Part print with two shaded views. Sizes in mm from the minimum x, y, z corner. Round coordinates to 2 decimals unless told otherwise and drop trailing zeros. Loops run counter-clockwise (first coordinate to the right, second up) from the corner with the lowest first, then second, coordinate; pieces in that order, holes last. Notation, with made-up numbers: M -27,46.25 L 18,46.25 A27 ccw 18,84.25 Z; hole C -31.75,34.25 d9. An arc over 180 degrees is marked long. Answer as CSV lines item,"result". Start each with the question number.
Item 1: Band-saw the part on A-A (x = 19.05). Give the cut face in (y, z), and give its area (3 significant figures).
Item 2: Mould opens along Z. For the marked faces 1, 2, 3 and 4 say: pulls with the +Z half, pulls with the -Z half, needs draft (parallel to the pull), parting line crosses it, or undercut.
Item 3: Band-saw the part on C-C (y = 3.5). Give the cut face in (x, z).
Item 4: Drop flat-ended pins along their axis: pin 1 Ø5 at (x, z) = (34.05, 34.05) entering from -Y; pin 2 Ø2 at (y, z) = (3.5, 15.5) entering from +X. Give the stop position or say it passes through.
Item 5: Wall check: line 1 (X direction, y = 5, z = 49.05); line 2 (X direction, y = 5, z = 9.5); line 3 (Z direction, x = 5, y = 1.25) (1 decimal). Give the ranges that are in metal, low to high.
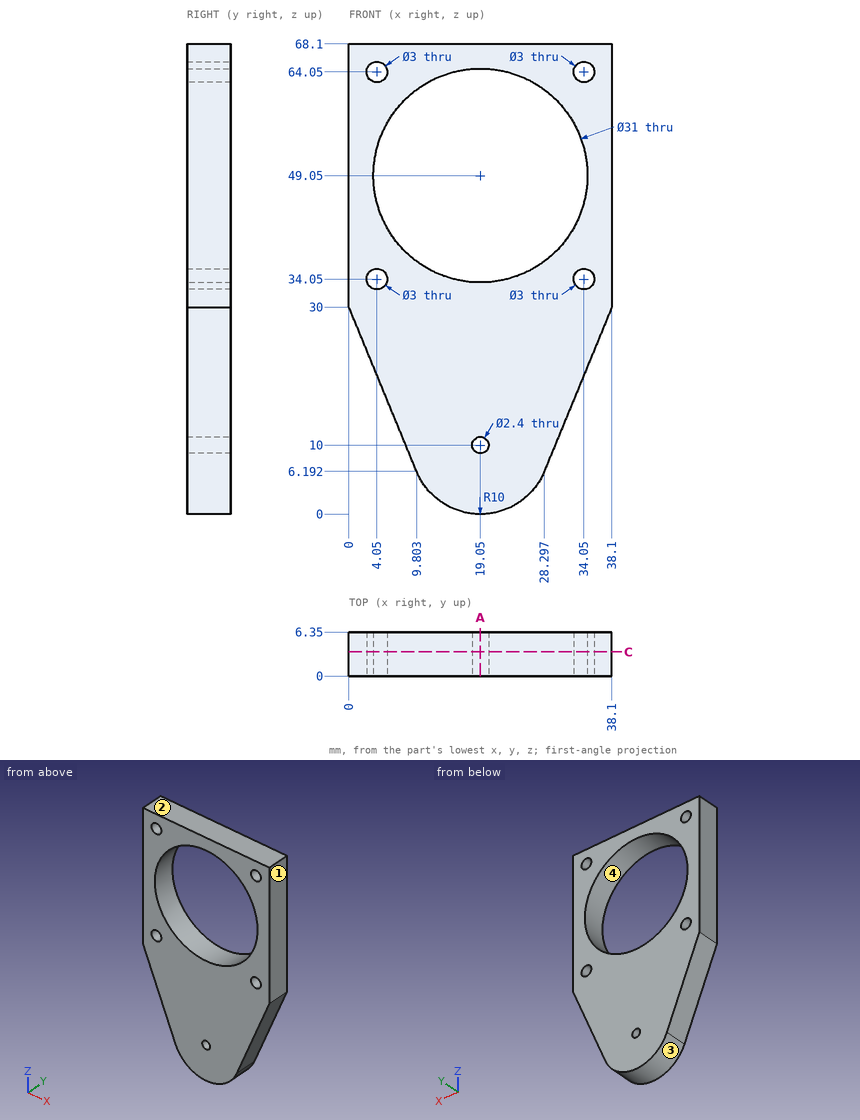
Answer block:
1,outline,"M 0,0 L 6.35,0 L 6.35,8.8 L 0,8.8 Z; M 0,11.2 L 6.35,11.2 L 6.35,33.55 L 0,33.55 Z; M 0,64.55 L 6.35,64.55 L 6.35,68.1 L 0,68.1 Z"
1,area,"220 mm^2"
2,face 1,"needs draft"
2,face 2,"pulls with the +Z half"
2,face 3,"pulls with the -Z half"
2,face 4,"undercut"
3,outline,"M 0,30 L 9.8,6.19 A10 ccw 28.3,6.19 L 38.1,30 L 38.1,68.1 L 0,68.1 Z; hole C 4.05,34.05 d3; hole C 4.05,64.05 d3; hole C 19.05,49.05 d31; hole C 19.05,10 d2.4; hole C 34.05,34.05 d3; hole C 34.05,64.05 d3"
4,pin 1,"stops at y = 0"
4,pin 2,"stops at x = 32.54"
5,line 1,"x = 0 to 3.55, 34.55 to 38.1"
5,line 2,"x = 8.44 to 17.96, 20.14 to 29.66"
5,line 3,"z = 17.9 to 32.9, 35.2 to 42.5, 55.6 to 62.9, 65.2 to 68.1"
